from build123d import *

# Parameters (mm, degrees)
F1_DEPTH  = 25.4
F3_DEPTH  = 25.4
F5_DEPTH  = 25.4
F6_R      = 6.5658374439
F7_DEPTH  = 25.4
F9_DEPTH  = 25.4
F11_DEPTH = 25.4
F13_DEPTH = 22.86


with BuildPart() as f1:
    # F0 (on Front) → F1 (new body)
    with BuildSketch(Plane.XZ):
        Polygon((0, 38.1), (0, 0), (69.85, 0), (69.85, 12.7), (19.05, 12.7), (19.05, 38.1), align=None)
    extrude(amount=F1_DEPTH)

    # F2 (on face) → F3 (cut)
    with BuildSketch(Plane.XY.offset(12.7)):
        with BuildLine():
            ThreePointArc((60.1857788861, 0), (67.0169340084, -4.8288024649), (69.85, -12.7))
            Line((69.85, -12.7), (69.85, 0))
            Line((69.85, 0), (60.1857788861, 0))
        make_face()
        with BuildLine():
            ThreePointArc((69.85, -12.7), (66.883728808, -20.4698334005), (60.1857788861, -25.4))
            Line((60.1857788861, -25.4), (69.85, -25.4))
            Line((69.85, -25.4), (69.85, -12.7))
        make_face()
    extrude(amount=-F3_DEPTH, mode=Mode.SUBTRACT)

    # F4 (on face) → F5 (cut)
    with BuildSketch(Plane.XY.offset(12.7)):
        with BuildLine():
            ThreePointArc((57.5700551271, -8.5117025301), (44.4156061858, -5.5470740223), (31.2611572444, -8.5117025301))
            ThreePointArc((31.2611572444, -8.5117025301), (29.3315874922, -12.6901739277), (31.2611572444, -16.8686453253))
            ThreePointArc((31.2611572444, -16.8686453253), (44.4156061858, -19.9707261196), (57.5700551271, -16.8686453253))
            ThreePointArc((57.5700551271, -16.8686453253), (59.9401679074, -12.6901739277), (57.5700551271, -8.5117025301))
        make_face()
    extrude(amount=-F5_DEPTH, mode=Mode.SUBTRACT)

    # F6 (on face) → F7 (cut)
    with BuildSketch(Plane.XY.offset(38.1)):
        with Locations((9.2854928225, -12.8449322656)):
            Circle(F6_R)
    extrude(amount=-F7_DEPTH, mode=Mode.SUBTRACT)

    # F8 (on face) → F9 (cut)
    with BuildSketch(Plane.XY.offset(38.1)):
        with BuildLine():
            ThreePointArc((9.525, 0), (18.786715691, -12.7), (9.525, -25.4))
            Line((9.525, -25.4), (19.05, -25.4))
            Line((19.05, -25.4), (19.05, 0))
            Line((19.05, 0), (9.525, 0))
        make_face()
    extrude(amount=-F9_DEPTH, mode=Mode.SUBTRACT)

    # F10 (on face) → F11 (cut)
    with BuildSketch(Plane.XY.offset(38.1)):
        with BuildLine():
            ThreePointArc((0, -11.9404586196), (2.7724235634, -4.3827293098), (9.525, 0))
            Line((9.525, 0), (0, 0))
            Line((0, 0), (0, -11.9404586196))
        make_face()
        with BuildLine():
            ThreePointArc((9.525, -25.4), (16.3361598408, -20.4049868588), (18.7813081047, -12.3202293098))
            ThreePointArc((18.7813081047, -12.3202293098), (15.1842035357, -21.293169718), (6.4328170235, -25.4))
            Line((6.4328170235, -25.4), (9.525, -25.4))
        make_face()
    extrude(amount=-F11_DEPTH, mode=Mode.SUBTRACT)

    # F12 (on face) → F13 (cut)
    with BuildSketch(Plane.XY.offset(38.1)):
        with BuildLine():
            ThreePointArc((6.4328170235, -25.4), (1.6908462088, -19.3993524556), (0, -11.9404586196))
            Line((0, -11.9404586196), (0, -25.4))
            Line((0, -25.4), (6.4328170235, -25.4))
        make_face()
    extrude(amount=-F13_DEPTH, mode=Mode.SUBTRACT)


solid = f1.part
Model file for the job. Use its own axes, mm. A direction names the side the tool comes from. Give positions to 0.01 mm unless a question says otherwise; leave off trailing zeros. Write each loop counter-clockwise with the first axis right and the second up, starting at its lowest first coordinate (ties: lowest second). Pieces come first, ordered by that corner, then holes. Notation, with made-up numbers: M -15.75,84 L 18.25,84 A19 cw 18.25,115 Z; hole C -28.5,76.5 d9. An arc over 180 degrees is marked long. One line per item, written item: value. Start each with the question number.
Q1. Saw through at B-B, the plane x = 59. Write the cut outline in (y, z).
Q2. Saw through at A-A, the plane z = 8.5. Write the cut outline in (x, y), plus the area to 3 significant figures.
Q3. Saw through at C-C, the plane y = -14.5. Write the cut outline in (x, z), plus the area to 3 significant figures.
Q4. Saw through at D-D, the plane x = 30.5. Write the cut outline in (y, z), plus the area to 3 significant figures.
Q5. Two-plate mould, pull along Y, no slides. Class faces 1 (the cylindrical face through (2.726, -12.556, 25.578)), 2 (the cylindrical face through (29.332, -12.624, 6.439)), 3 (the cylindrical face through (66.95, -20.38, 6.44)), 4 (the cylindrical face through (16.043, -4.596, 25.578)): +Y half, -Y half, draft (parallel to the pull), parting line (faces both ways), or undercut.
Q6. Drop flat-ended pins along their axis: pin 1 Ø1 at (x, y) = (47.5, -7) entering from +Z; pin 2 Ø1.5 at (x, y) = (23, -7) entering from +Z; pin 3 Ø8 at (y, z) = (-17, 15) entering from +X. Give the stop position or say it passes through.
Q7. Probe probe 1 along Z at (x, y) = (21, -16.75); probe 2 along X at (y, z) = (-16.5, 9.5); probe 3 along Y at (x, z) = (11, 17). List the from-to ranges inside material, lowest first. Write a range as [from, to].
Q8. 3-axis set-ups, long thin cutter, end or side, ignore diameter. For faces 5 (the cylindrical face through (2.701, -4.473, 25.578)), 6 (the flat face through (9, -13, 12.7)), 7 (the cylindrical face through (15.28, -21.19, 25.58)), 8 (the cylindrical face through (44.606, -5.548, 6.439)): which of +Z, -Z, +X, -X, +Y, -Y reach the whole face in a straight line?
Output values:
1. outline: M -25.4,0 L -15.57,0 L -15.57,12.7 L -25.4,12.7 Z; M -9.81,0 L 0,0 L 0,12.7 L -9.81,12.7 Z
2. outline: M 0,-25.4 L 60.19,-25.4 A14.75 ccw 69.85,-12.7 A13.93 ccw 60.19,0 L 0,0 Z; hole M 31.26,-16.87 A29.44 ccw 57.57,-16.87 A4.87 ccw 57.57,-8.51 A30.67 ccw 31.26,-8.51 A5.49 ccw Z
2. area: 1,350 mm²
3. outline: M 0,0 L 29.64,0 L 29.64,12.7 L 18.59,12.7 L 18.59,38.1 L 15.64,38.1 L 15.64,12.7 L 2.93,12.7 L 2.93,38.1 L 0.19,38.1 L 0.19,15.24 L 0,15.24 Z; M 59.59,0 L 69.6,0 L 69.6,12.7 L 59.59,12.7 Z
3. area: 648 mm²
4. outline: M -25.4,0 L -16.08,0 L -16.08,12.7 L -25.4,12.7 Z; M -9.3,0 L 0,0 L 0,12.7 L -9.3,12.7 Z
4. area: 237 mm²
5. face 1: undercut
5. face 2: undercut
5. face 3: -Y half
5. face 4: +Y half
6. pin 1: passes through
6. pin 2: stops at z = 12.7
6. pin 3: stops at x = 69.73
7. probe 1: z = [0, 12.7]
7. probe 2: x = [0, 30.87], [58.1, 69.04]
7. probe 3: y = [-24.27, -19.18], [-6.51, -0.57]
8. face 5: +Z, -X, +Y
8. face 6: +Z
8. face 7: +Z, +X, -Y
8. face 8: +Z, -Z
